from build123d import *

# Parameters (mm, degrees)
F0_W      = 5.108088
F0_H      = 4.79851
F1_DEPTH  = 4.5
F2_W      = 6.587152
F2_H      = 6.533596
F6_DEPTH  = 5.5
F3_W      = 4.659206
F3_H      = 3.320352
F7_DEPTH  = 3.5
F4_W      = 4.070107
F4_H      = 6.747813
F9_DEPTH  = 4
F5_W      = 4.284326
F5_H      = 4.123662
F10_DEPTH = 2.5
F8_W      = 4.406571
F8_H      = 5.095096
F11_DEPTH = 4.5
F12_R     = 0.503624
F13_DEPTH = 3.5


with BuildPart() as f1:
    # F0 (on Front) → F1 (new body)
    with BuildSketch(Plane.XZ):
        with Locations((-50.157245, 31.105429)):
            Rectangle(F0_W, F0_H)
    extrude(amount=F1_DEPTH)

    # F2 (on Front) → F6 (join)
    with BuildSketch(Plane.XZ):
        with Locations((-46.830697, 28.015254)):
            Rectangle(F2_W, F2_H)
    extrude(amount=F6_DEPTH)

    # F3 (on Front) → F7 (join)
    with BuildSketch(Plane.XZ):
        with Locations((-51.489901, 28.068807)):
            Rectangle(F3_W, F3_H)
    extrude(amount=F7_DEPTH)

    # F4 (on Front) → F9 (join)
    with BuildSketch(Plane.XZ):
        with Locations((-50.177825, 24.212915)):
            Rectangle(F4_W, F4_H)
    extrude(amount=F9_DEPTH)

    # F5 (on Front) → F10 (join)
    with BuildSketch(Plane.XZ):
        with Locations((-47.23235, 23.704151)):
            Rectangle(F5_W, F5_H)
    extrude(amount=F10_DEPTH)

    # F8 (on Front) → F11 (join)
    with BuildSketch(Plane.XZ):
        with Locations((-47.829266, 20.953265)):
            Rectangle(F8_W, F8_H)
    extrude(amount=F11_DEPTH)

    # F12 (on face) → F13 (cut)
    with BuildSketch(Plane.XY.offset(33.504684)):
        with Locations((-49.100351, -2.427287)):
            Circle(F12_R)
    extrude(amount=-F13_DEPTH, mode=Mode.SUBTRACT)


solid = f1.part
Geometry check sheet. Reference: the model listing, model coordinates, mm. A direction names the side the tool comes from. Give positions to 0.01 mm unless a question says otherwise; leave off trailing zeros. Loops run counter-clockwise (first coordinate to the right, second up) from the corner with the lowest first, then second, coordinate; pieces in that order, holes last.
(1) Section check B-B on x = -46. Record the cut outline in (y, z), then the cut area to 3 significant figures.
From the geometry:
outline: (-5.5, 24.75) - (-2.5, 24.75) - (-2.5, 23.5) - (-4.5, 23.5) - (-4.5, 18.41) - (0, 18.41) - (0, 31.28) - (-5.5, 31.28) - close
area: 62.0 mm2
(2) Section check D-D on z = 24.25. Record the cut outline in (x, y).
From the geometry:
outline: (-52.21, -4) - (-48.14, -4) - (-48.14, -2.5) - (-45.09, -2.5) - (-45.09, 0) - (-52.21, 0) - close
(3) Set-up check for faces 1 (the flat face through (-51, -4, 28.706)), 2 (the flat face through (-47.603, -2, 32)), 3 (the flat face through (-45.09, -1, 23)), 4 (the flat face through (-48.143, -3, 24)): record each of +Z, -Z, +X, -X, +Y, -Y from which the full face is reachable in a straight line by a thin tool's end or side.
From the geometry:
face 1: -X, -Y
face 2: +Z, +X, +Y, -Y
face 3: -Z, +X, +Y, -Y
face 4: +X, -Y
(4) Section check C-C on z = 30.5. Record the cut outline in (x, y), then the cut area to 3 significant figures.
From the geometry:
outline: (-52.71, -4.5) - (-50.12, -4.5) - (-50.12, -5.5) - (-43.54, -5.5) - (-43.54, 0) - (-52.71, 0) - close; hole circle Ø1.01 at (-49.1, -2.43)
area: 47.1 mm2
(5) Depth check by flat-ended pin: pin 1 Ø1.2 at (x, y) = (-53.5, -2) entering from +Z; pin 2 Ø1.5 at (x, z) = (-47.5, 20.5) entering from -Y; pin 3 Ø1 at (x, z) = (-52, 27.5) entering from -Y. Enter the tip coordinate at first touch or a pass-through.
From the geometry:
pin 1: stops at z = 29.73
pin 2: stops at y = -4.5
pin 3: stops at y = -4
(6) Section check A-A on y = -4.25. Record the cut outline in (x, z).
From the geometry:
outline: (-52.71, 28.71) - (-50.12, 28.71) - (-50.12, 24.75) - (-43.54, 24.75) - (-43.54, 31.28) - (-47.6, 31.28) - (-47.6, 33.5) - (-52.71, 33.5) - close; (-50.03, 18.41) - (-45.63, 18.41) - (-45.63, 23.5) - (-50.03, 23.5) - close
(7) Release check for a two-part mould opening along Z. For faces 5 (the flat face through (-46, -2.5, 24)), 6 (the flat face through (-48, -4.5, 21)), 7 (the flat face through (-53, -2, 26.409)) record: released by +Z, released by -Z, zero draft, split by the parting line, or undercut.
From the geometry:
face 5: undercut
face 6: zero draft
face 7: released by -Z
(8) Thickness scan on L1, parallel to Z at x = -46.25, y = -4.05; L2, parallel to Z at x = -48, y = -3.05; L3, parallel to Y at x = -48.25, z = 24.5. Record the ranges inside material, lowest first.
From the geometry:
L1: z = 18.41 to 23.5, 24.75 to 31.28
L2: z = 18.41 to 23.5, 24.75 to 33.5
L3: y = -4 to 0
